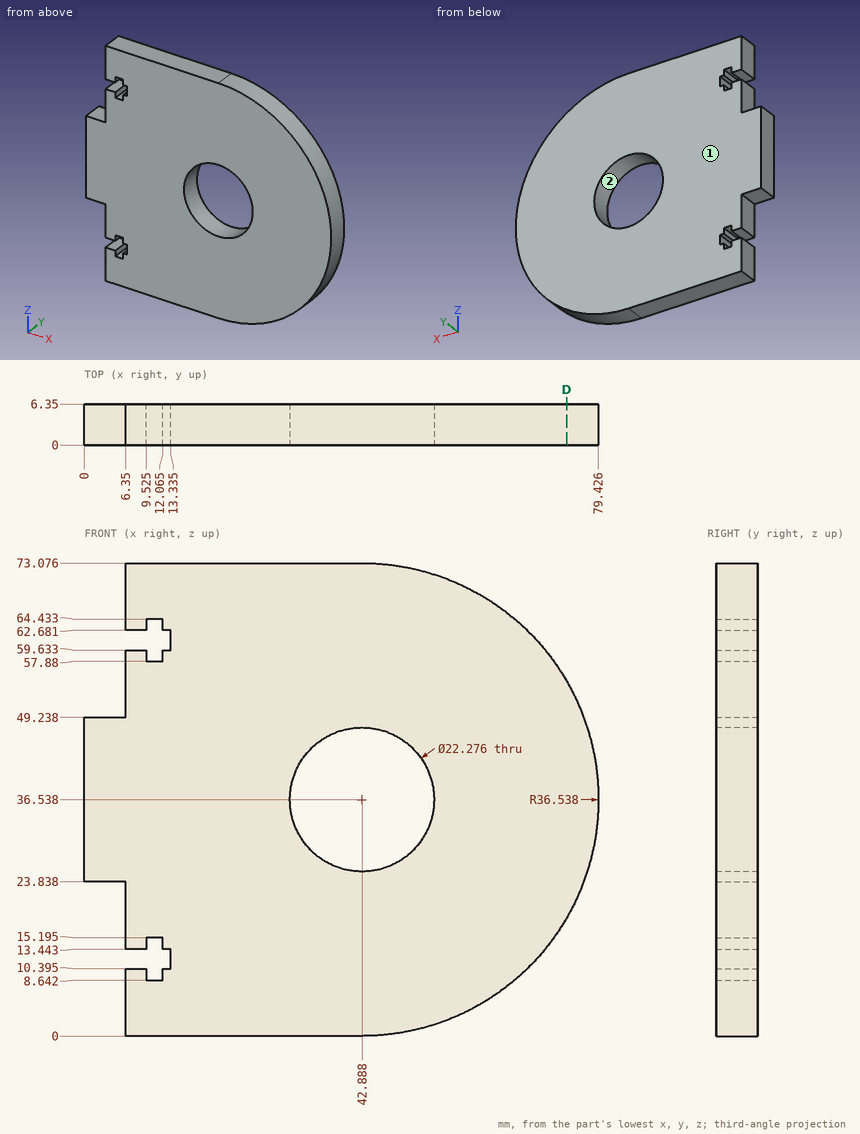
Could you check a few things on this drawing? It's one solid part, dimensions in mm from its lowest x, y, z. Round coordinates to 2 decimals unless told otherwise and drop trailing zeros. Loops run counter-clockwise (first coordinate to the right, second up) from the corner with the lowest first, then second, coordinate; pieces in that order, holes last. Notation, with made-up numbers: (25, 77) -> (50, 77) arc R7 ccw to (50, 89) -> close; hole circle Ø6 at (60, 43). An arc over 180 degrees is marked (long way). Write each question's results on one line, items separated by ' | '.
(1) For P1, Ø1.4, axis at y = 2, z = 9.5, coming from the -X side; P2, Ø0.5, axis at y = 2.5, z = 14, coming from the +X side; P3, Ø1.9, axis at y = 1.5, z = 9.5, coming from the +X side, each with a flat end and sliding along its axis, tell me the tip position at first contact or that it passes through.
Worked answers:
P1: x = 6.35 | P2: x = 71.84 | P3: x = 68.47
(2) We'd pull the mould along Z, two halves only. Please class the marked faces 1 and 2: released by +Z, released by -Z, zero draft, split by the parting line, or undercut.
Worked answers:
face 1: zero draft | face 2: undercut
(3) If I drill on L1, parallel to Z at x = 7.5, y = 2.5 (1 decimal); L2, parallel to Z at x = 42.5, y = 5.5 (1 decimal); L3, parallel to X at y = 5.75, z = 43.5 (1 decimal), over which ranges is the centre line in solid material (lowest first)?
Worked answers:
L1: 0 to 10.4, 13.4 to 59.6, 62.7 to 73.1 | L2: 0 to 25.4, 47.7 to 73.1 | L3: 0 to 34.2, 51.6 to 78.8
(4) If we section it at D-D, the plane x = 74.5: List the corners of the cut face in (y, z) for me, then the cut area to 3 significant figures.
Worked answers:
outline: (0, 18.22) -> (6.35, 18.22) -> (6.35, 54.86) -> (0, 54.86) -> close | area: 233 mm2
